Verification items for the finished model (mm, model axes). Round coordinates to 2 decimals unless told otherwise and drop trailing zeros. Write each loop counter-clockwise with the first axis right and the second up, starting at its lowest first coordinate (ties: lowest second). Pieces come first, ordered by that corner, then holes.
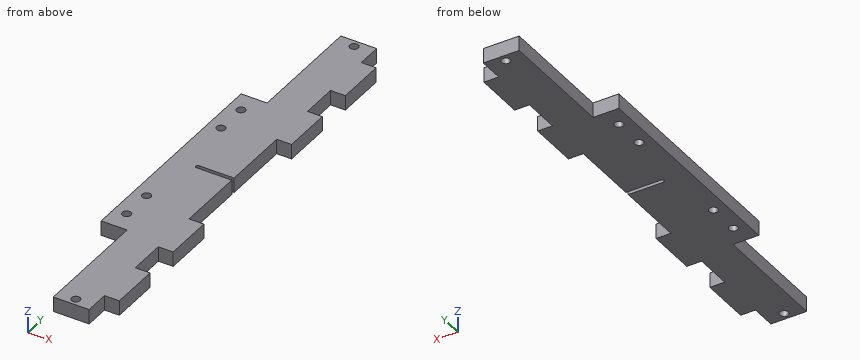
from build123d import *

# Parameters (mm, degrees)
ESBO_O1_W                = 10.5
ESBO_O1_H                = 91
RESSALTO_EXTRUS_O1_DEPTH = 6
ESBO_O2_W                = 6
ESBO_O2_H                = 20
RESSALTO_EXTRUS_O2_DEPTH = 6
ESBO_O3_R                = 1.75
CORTE_EXTRUS_O2_DEPTH    = 25.5
ESBO_O4_W                = 15
ESBO_O4_H                = 1.5
CORTE_EXTRUS_O3_DEPTH    = 6
FILETE1_R                = 0.75
ESBO_O5_R                = 1.75
CORTE_EXTRUS_O4_DEPTH    = 6


with BuildPart() as part:
    # Esboço1 → Ressalto-extrusão1 (new body)
    with BuildSketch(Plane.XY):
        with Locations((98.05, -93.5)):
            Rectangle(ESBO_O1_W, ESBO_O1_H)
        Polygon((117.8, 0), (103.3, 0), (103.3, -48), (103.3, -139), (103.3, -187), (117.8, -187), align=None)
    extrude(amount=-RESSALTO_EXTRUS_O1_DEPTH)

    # Esboço2 → Ressalto-extrusão2 (add)
    with BuildSketch(Plane.XY):
        with Locations((120.8, -20)):
            Rectangle(ESBO_O2_W, ESBO_O2_H)
        with Locations((120.8, -55)):
            Rectangle(ESBO_O2_W, ESBO_O2_H)
    ressalto_extrus_o2 = extrude(amount=-RESSALTO_EXTRUS_O2_DEPTH)

    # Espelhar1: Ressalto-extrusão2 across plane
    add(ressalto_extrus_o2.mirror(Plane.ZX.offset(-93.5)))

    # Esboço3 → Corte-extrusão2 (cut)
    with BuildSketch(Plane.XY):
        with Locations((97.95, -56.3)):
            Circle(ESBO_O3_R)
        with Locations((97.95, -69.3)):
            Circle(ESBO_O3_R)
        with Locations((97.95, -117.7)):
            Circle(ESBO_O3_R)
        with Locations((97.95, -130.7)):
            Circle(ESBO_O3_R)
    extrude(amount=-CORTE_EXTRUS_O2_DEPTH, mode=Mode.SUBTRACT)

    # Esboço4 → Corte-extrusão3 (cut)
    with BuildSketch(Plane.XY):
        with Locations((110.3, -93.5)):
            Rectangle(ESBO_O4_W, ESBO_O4_H)
    extrude(amount=-CORTE_EXTRUS_O3_DEPTH, mode=Mode.SUBTRACT)

    # Filete1
    filete1_edges = [part.edges().sort_by_distance(p)[0] for p in [
        (102.8, -94.25, -3),
        (102.8, -92.75, -3),
    ]]
    fillet(filete1_edges, radius=FILETE1_R - 0.0001)  # a hair under: the kernel refuses the full size

    # Esboço5 → Corte-extrusão4 (cut)
    with BuildSketch(Plane.XY):
        with Locations((110.55, -184)):
            Circle(ESBO_O5_R)
    corte_extrus_o4 = extrude(amount=-CORTE_EXTRUS_O4_DEPTH, mode=Mode.SUBTRACT)

    # Espelhar2: Corte-extrusão4 across plane
    add(corte_extrus_o4.mirror(Plane.ZX.offset(-93.5)), mode=Mode.SUBTRACT)


solid = part.part
Q1. Sectioned sample at C-C (x = 97.95). Enter the section's corners in (y, z).
Recorded:
outline: (-139, -6) - (-132.45, -6) - (-132.45, 0) - (-139, 0) - close; (-128.95, -6) - (-119.45, -6) - (-119.45, 0) - (-128.95, 0) - close; (-115.95, -6) - (-71.05, -6) - (-71.05, 0) - (-115.95, 0) - close; (-67.55, -6) - (-58.05, -6) - (-58.05, 0) - (-67.55, 0) - close; (-54.55, -6) - (-48, -6) - (-48, 0) - (-54.55, 0) - close
Q2. Material ranges on line 1 along Y through (x, z) = (110.55, -3.2); line 2 along Y through (x, z) = (120.5, -2.4); line 3 along Y through (x, z) = (113, -1.6), recorded low to high.
Recorded:
line 1: y = -187 to -185.75, -182.25 to -94.25, -92.75 to -4.75, -1.25 to 0
line 2: y = -177 to -157, -142 to -122, -65 to -45, -30 to -10
line 3: y = -187 to -94.25, -92.75 to 0
Q3. Depth check by flat-ended pin: P1, Ø1.8, axis at x = 120, z = -3, coming from the +Y side; P2, Ø3, axis at x = 121, z = -3, coming from the -Y side; P3, Ø3, axis at y = -154.5, z = -3, coming from the -X side. Enter the tip coordinate at first touch or a pass-through.
Recorded:
P1: stops at y = -10
P2: stops at y = -177
P3: stops at x = 103.3
Q4. Sectioned sample at D-D (y = -184). Enter the section's corners in (x, z).
Recorded:
outline: (103.3, -6) - (108.8, -6) - (108.8, 0) - (103.3, 0) - close; (112.3, -6) - (117.8, -6) - (117.8, 0) - (112.3, 0) - close
Q5. Sectioned sample at A-A (y = -117.7). Enter the section's corners in (x, z), plus the area to 3 significant figures.
Recorded:
outline: (92.8, -6) - (96.2, -6) - (96.2, 0) - (92.8, 0) - close; (99.7, -6) - (117.8, -6) - (117.8, 0) - (99.7, 0) - close
area: 129 mm2
Q6. Sectioned sample at B-B (x = 122). Enter the section's corners in (y, z), plus the area to 3 significant figures.
Recorded:
outline: (-177, -6) - (-157, -6) - (-157, 0) - (-177, 0) - close; (-142, -6) - (-122, -6) - (-122, 0) - (-142, 0) - close; (-65, -6) - (-45, -6) - (-45, 0) - (-65, 0) - close; (-30, -6) - (-10, -6) - (-10, 0) - (-30, 0) - close
area: 480 mm2
